Verification items for this drawing (mm, ordinates from the low corner). Round coordinates to 2 decimals unless told otherwise and drop trailing zeros. Order: outer loops, then holes, each group sorted by start corner. A loop starts at its lowest first (then second) coordinate and runs counter-clockwise, first axis right, second up.
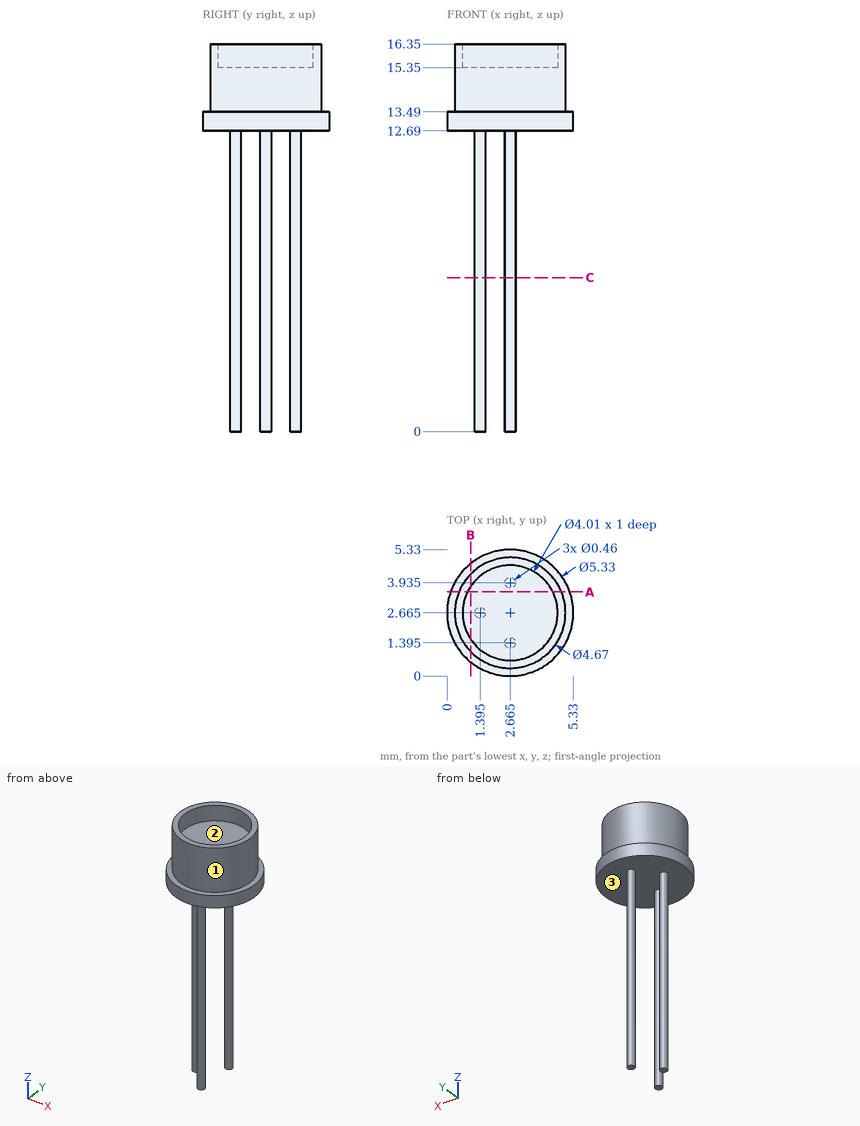
Item 1: Sectioned sample at A-A (y = 3.55). Record the cut outline in (x, z).
Answer:
outline: (0.15, 12.69) - (5.18, 12.69) - (5.18, 13.49) - (4.83, 13.49) - (4.83, 16.35) - (4.46, 16.35) - (4.46, 15.35) - (0.87, 15.35) - (0.87, 16.35) - (0.5, 16.35) - (0.5, 13.49) - (0.15, 13.49) - close
Item 2: Sectioned sample at B-B (x = 1). Record the cut outline in (y, z).
Answer:
outline: (0.58, 12.69) - (4.75, 12.69) - (4.75, 13.49) - (4.3, 13.49) - (4.3, 16.35) - (3.78, 16.35) - (3.78, 15.35) - (1.55, 15.35) - (1.55, 16.35) - (1.03, 16.35) - (1.03, 13.49) - (0.58, 13.49) - close
Item 3: Sectioned sample at C-C (z = 6.5). Record the cut outline in (x, y) (3 decimals).
Answer:
outline: circle Ø0.46 at (1.395, 2.665); circle Ø0.46 at (2.665, 1.395); circle Ø0.46 at (2.665, 3.935)
Item 4: Release check for a two-part mould opening along X. For the marked faces 1, 2 and 3 record: released by +X, released by -X, zero draft, split by the parting line, or undercut.
Answer:
face 1: split by the parting line
face 2: undercut
face 3: zero draft
Item 5: Scan lines: line 1 along Z through (x, y) = (3.6, 3.5); line 2 along Z through (x, y) = (2.3, 4.8); line 3 along Y through (x, z) = (1.65, 15.5). Record each from-to range of solid material in increasing order.
Answer:
line 1: z = 12.69 to 15.35
line 2: z = 12.69 to 16.35
line 3: y = 0.56 to 0.94, 4.39 to 4.77
Item 6: Go/stop test with flat-tipped pins: P1, Ø3, axis at x = 2.5, y = 3.5, coming from the +Z side; P2, Ø1, axis at x = 3.5, y = 2.5, coming from the +Z side; P3, Ø1.5, axis at x = 5, z = 13, coming from the -Y side. Record where each tip stops, or that it passes through.
Answer:
P1: stops at z = 16.35
P2: stops at z = 15.35
P3: stops at y = 0.52
